from build123d import *

# Parameters (mm, degrees)
BOSS_EXTRUDE1_DEPTH = 6.35
CUT_EXTRUDE1_START  = -6.35
CUT_EXTRUDE1_DEPTH  = 6.35


with BuildPart() as part:
    # Model → Boss-Extrude1 (new body)
    with BuildSketch(Plane.XY):
        Polygon((-95.25, 386.08), (-6.35, 386.08), (-6.35, 436.88), (0, 436.88), (0, 0), (-101.6, 0), (-101.6, 436.88), (-95.25, 436.88), align=None)
        with BuildLine():
            Line((-80.76878597, 311.15), (-12.7, 311.15))
            ThreePointArc((-12.7, 311.15), (-8.209871939, 313.009871939), (-6.35, 317.5))
            Line((-6.35, 317.5), (-6.35, 363.45223644))
            ThreePointArc((-6.35, 363.45223644), (-7.711169032, 365.702115893), (-10.335793346, 365.540604607))
            Line((-10.335793346, 365.540604607), (-82.214579316, 315.778368167))
            ThreePointArc((-82.214579316, 315.778368167), (-83.193250358, 312.932654354), (-80.76878597, 311.15))
        make_face(mode=Mode.SUBTRACT)
        with BuildLine():
            Line((-95.25, 287.25223644), (-95.25, 241.3))
            ThreePointArc((-95.25, 241.3), (-93.390128061, 236.809871939), (-88.9, 234.95))
            Line((-88.9, 234.95), (-20.83121403, 234.95))
            ThreePointArc((-20.83121403, 234.95), (-18.406749642, 236.732654354), (-19.385420684, 239.578368167))
            Line((-19.385420684, 239.578368167), (-91.264206654, 289.340604607))
            ThreePointArc((-91.264206654, 289.340604607), (-93.888830968, 289.502115893), (-95.25, 287.25223644))
        make_face(mode=Mode.SUBTRACT)
        with BuildLine():
            Line((-80.76878597, 158.75), (-12.7, 158.75))
            ThreePointArc((-12.7, 158.75), (-8.209871939, 160.609871939), (-6.35, 165.1))
            Line((-6.35, 165.1), (-6.35, 211.05223644))
            ThreePointArc((-6.35, 211.05223644), (-7.711169032, 213.302115893), (-10.335793346, 213.140604607))
            Line((-10.335793346, 213.140604607), (-82.214579316, 163.378368167))
            ThreePointArc((-82.214579316, 163.378368167), (-83.193250358, 160.532654354), (-80.76878597, 158.75))
        make_face(mode=Mode.SUBTRACT)
        with BuildLine():
            Line((-20.83121403, 222.25), (-88.9, 222.25))
            ThreePointArc((-88.9, 222.25), (-93.390128061, 220.390128061), (-95.25, 215.9))
            Line((-95.25, 215.9), (-95.25, 169.94776356))
            ThreePointArc((-95.25, 169.94776356), (-93.888830968, 167.697884107), (-91.264206654, 167.859395393))
            Line((-91.264206654, 167.859395393), (-19.385420684, 217.621631833))
            ThreePointArc((-19.385420684, 217.621631833), (-18.406749642, 220.467345646), (-20.83121403, 222.25))
        make_face(mode=Mode.SUBTRACT)
        with BuildLine():
            Line((-82.214579316, 293.821631833), (-10.335793346, 244.059395393))
            ThreePointArc((-10.335793346, 244.059395393), (-7.711169032, 243.897884107), (-6.35, 246.14776356))
            Line((-6.35, 246.14776356), (-6.35, 292.1))
            ThreePointArc((-6.35, 292.1), (-8.209871939, 296.590128061), (-12.7, 298.45))
            Line((-12.7, 298.45), (-80.76878597, 298.45))
            ThreePointArc((-80.76878597, 298.45), (-83.193250358, 296.667345646), (-82.214579316, 293.821631833))
        make_face(mode=Mode.SUBTRACT)
        with BuildLine():
            Line((-95.25, 134.85223644), (-95.25, 88.9))
            ThreePointArc((-95.25, 88.9), (-93.390128061, 84.409871939), (-88.9, 82.55))
            Line((-88.9, 82.55), (-20.83121403, 82.55))
            ThreePointArc((-20.83121403, 82.55), (-18.406749642, 84.332654354), (-19.385420684, 87.178368167))
            Line((-19.385420684, 87.178368167), (-91.264206654, 136.940604607))
            ThreePointArc((-91.264206654, 136.940604607), (-93.888830968, 137.102115893), (-95.25, 134.85223644))
        make_face(mode=Mode.SUBTRACT)
        with BuildLine():
            Line((-80.76878597, 6.35), (-12.7, 6.35))
            ThreePointArc((-12.7, 6.35), (-8.209871939, 8.209871939), (-6.35, 12.7))
            Line((-6.35, 12.7), (-6.35, 58.65223644))
            ThreePointArc((-6.35, 58.65223644), (-7.711169032, 60.902115893), (-10.335793346, 60.740604607))
            Line((-10.335793346, 60.740604607), (-82.214579316, 10.978368167))
            ThreePointArc((-82.214579316, 10.978368167), (-83.193250358, 8.132654354), (-80.76878597, 6.35))
        make_face(mode=Mode.SUBTRACT)
        with BuildLine():
            Line((-20.83121403, 69.85), (-88.9, 69.85))
            ThreePointArc((-88.9, 69.85), (-93.390128061, 67.990128061), (-95.25, 63.5))
            Line((-95.25, 63.5), (-95.25, 17.54776356))
            ThreePointArc((-95.25, 17.54776356), (-93.888830968, 15.297884107), (-91.264206654, 15.459395393))
            Line((-91.264206654, 15.459395393), (-19.385420684, 65.221631833))
            ThreePointArc((-19.385420684, 65.221631833), (-18.406749642, 68.067345646), (-20.83121403, 69.85))
        make_face(mode=Mode.SUBTRACT)
        with BuildLine():
            Line((-20.83121403, 374.65), (-88.9, 374.65))
            ThreePointArc((-88.9, 374.65), (-93.390128061, 372.790128061), (-95.25, 368.3))
            Line((-95.25, 368.3), (-95.25, 322.34776356))
            ThreePointArc((-95.25, 322.34776356), (-93.888830968, 320.097884107), (-91.264206654, 320.259395393))
            Line((-91.264206654, 320.259395393), (-19.385420684, 370.021631833))
            ThreePointArc((-19.385420684, 370.021631833), (-18.406749642, 372.867345646), (-20.83121403, 374.65))
        make_face(mode=Mode.SUBTRACT)
        with BuildLine():
            Line((-82.214579316, 141.421631833), (-10.335793346, 91.659395393))
            ThreePointArc((-10.335793346, 91.659395393), (-7.711169032, 91.497884107), (-6.35, 93.74776356))
            Line((-6.35, 93.74776356), (-6.35, 139.7))
            ThreePointArc((-6.35, 139.7), (-8.209871939, 144.190128061), (-12.7, 146.05))
            Line((-12.7, 146.05), (-80.76878597, 146.05))
            ThreePointArc((-80.76878597, 146.05), (-83.193250358, 144.267345646), (-82.214579316, 141.421631833))
        make_face(mode=Mode.SUBTRACT)
    extrude(amount=BOSS_EXTRUDE1_DEPTH)

    # Sketch1 → Cut-Extrude1 (cut)
    with BuildSketch(Plane.XY.offset(6.35).offset(CUT_EXTRUDE1_START)):
        with BuildLine():
            Line((-12.7, 82.55), (-88.9, 82.55))
            ThreePointArc((-88.9, 82.55), (-93.390128061, 84.409871939), (-95.25, 88.9))
            Line((-95.25, 88.9), (-95.25, 215.9))
            ThreePointArc((-95.25, 215.9), (-93.390128061, 220.390128061), (-88.9, 222.25))
            Line((-88.9, 222.25), (-12.7, 222.25))
            ThreePointArc((-12.7, 222.25), (-8.209871939, 220.390128061), (-6.35, 215.9))
            Line((-6.35, 215.9), (-6.35, 88.9))
            ThreePointArc((-6.35, 88.9), (-8.209871939, 84.409871939), (-12.7, 82.55))
        make_face()
    extrude(amount=CUT_EXTRUDE1_DEPTH, mode=Mode.SUBTRACT)


solid = part.part
Build history of the part. All positions in model axes, mm. A direction names the side the tool comes from. Round coordinates to 2 decimals unless told otherwise and drop trailing zeros. Write each loop counter-clockwise with the first axis right and the second up, starting at its lowest first coordinate (ties: lowest second). Pieces come first, ordered by that corner, then holes. Notation, with made-up numbers: M 38,19.25 L 70,19.25 A33 ccw 70,52.25 Z; hole C -38,68.5 d10. An arc over 180 degrees is marked long. Answer as a JSON object with one key per item and string values. Group by question number.
(1) Cut at A-A (y = 128). Give the cut face in (x, z).
(2) Drill centre lines: L1, parallel to X at y = 193, z = 2.25; L2, parallel to X at y = 26.5, z = 2; L3, parallel to X at y = 21, z = 2. Where is each one in solid material? Low to high.
(3) Cut at D-D (y = 269). Give the cut face in (x, z).
(4) Mould opens along X. For faces 1 (the flat face through (-46.78, 269.29, 3.13)), 2 (the flat face through (-36, 252, 0)) say: pulls with the +X half, pulls with the -X half, needs draft (parallel to the pull), parting line crosses it, or undercut.
(5) Cut at B-B (x = -35). Give the number of separate pieces and of enclosed holes in the cut face, and give its area (3 significant figures).
(6) Which spindle directions (+Z, -Z, +X, -X, +Y, -Y) get a long thin tool onto all of the face, cutting with end or side? Do faces 3 (the flat face through (-55.83, 344.79, 3.13)), 4 (the flat face through (-36, 252, 6.35)). Say none if no direction does.
(7) Flat gauge pin, fed straight in: pin 1 (3 mm diameter, centred on x = -65.5, z = 2, fed in from +Y). Where does the tip first touch, or does it go through?
Responses:
{
 "1": {"outline": "M -101.6,0 L -95.25,0 L -95.25,6.35 L -101.6,6.35 Z; M -6.35,0 L 0,0 L 0,6.35 L -6.35,6.35 Z"},
 "2": {"L1": "x = -101.6 to -95.25, -6.35 to 0", "L2": "x = -101.6 to -95.25, -75.32 to -59.79, -6.35 to 0", "L3": "x = -101.6 to -95.25, -83.26 to -67.74, -6.35 to 0"},
 "3": {"outline": "M -101.6,0 L -95.25,0 L -95.25,6.35 L -101.6,6.35 Z; M -61.88,0 L -46.36,0 L -46.36,6.35 L -61.88,6.35 Z; M -6.35,0 L 0,0 L 0,6.35 L -6.35,6.35 Z"},
 "4": {"face 1": "undercut", "face 2": "needs draft"},
 "5": {"separate pieces": "8", "enclosed holes": "0", "area": "560 mm2"},
 "6": {"face 3": "+Z, -Z", "face 4": "+Z, +X, -X, +Y, -Y"},
 "7": {"pin 1": "stops at y = 386.08"}
}
